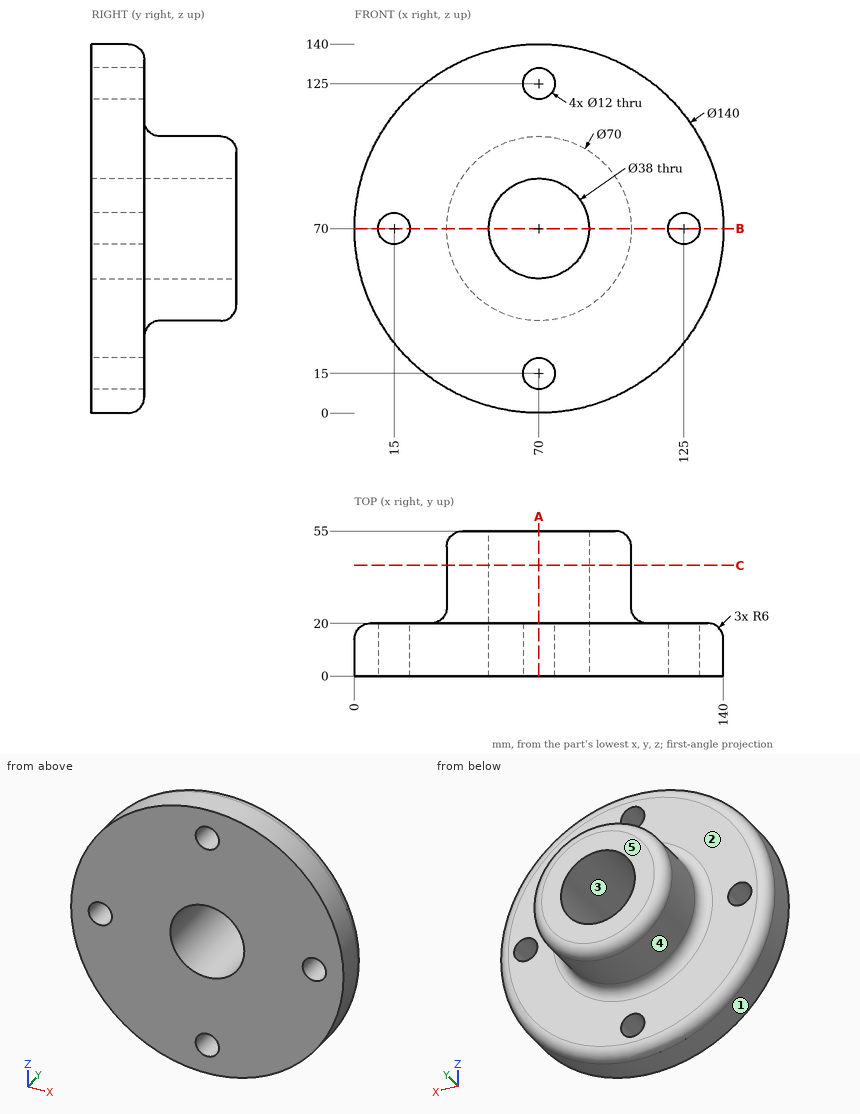
Could you check a few things on this drawing? It's one solid part, dimensions in mm from its lowest x, y, z. A direction names the side the tool comes from. Coordinates: 2 decimals unless noted, no trailing zeros. Loops run counter-clockwise (first coordinate to the right, second up) from the corner with the lowest first, then second, coordinate; pieces in that order, holes last. Notation, with made-up numbers: (67.5, -34.75) - (104.5, -34.75) arc R29 cw to (104.5, -2.75) - close; hole circle Ø7 at (-37, -37). An arc over 180 degrees is marked (long way). Answer as a JSON object with one key per item and string values. Group by question number.
Item 1: For pin 1 (9.5 mm diameter, centred on x = 125, z = 70, fed in from +Y); pin 2 (1.5 mm diameter, centred on x = 41, z = 47, fed in from +Y); pin 3 (2 mm diameter, centred on y = 10, z = 38.5, fed in from +X); pin 4 (2 mm diameter, centred on y = 13.5, z = 76, fed in from -X), each with a flat end and sliding along its axis, tell me the tip position at first contact or that it passes through.
Item 2: If I drill on L1, parallel to Z at x = 70, y = 12; L2, parallel to Z at x = 70, y = 38; L3, parallel to Y at x = 34, z = 119, over which ranges is the centre line in solid material (lowest first)? Write a range as from..to.
Item 3: If we section it at C-C (y = 42): List the corners of the cut face in (x, z) for me.
Item 4: On a 3-axis mill with a long thin cutter (end or side, diameter ignored), from which of +Z, -Z, +X, -X, +Y, -Y can I reach the whole of each face in a straight line? I mean the marked faces 4 and 5. Say none if no direction works.
Item 5: If we section it at B-B (z = 70): List the corners of the cut face in (x, y) for me.
Item 6: If we mould it in two halves opening along Z, with no side actions, what happens to the marked faces 1, 2 and 3? For each: released by +Z, released by -Z, zero draft, split by the parting line, or undercut.
Item 7: If we section it at A-A (x = 70): List the corners of the cut face in (y, z) for me.
Returned:
{
 "1": {"pin 1": "passes through", "pin 2": "stops at y = 22.32", "pin 3": "stops at x = 133.01", "pin 4": "stops at x = 0.18"},
 "2": {"L1": "z = 0..9, 21..51, 89..119, 131..140", "L2": "z = 35..51, 89..105", "L3": "y = 0..20"},
 "3": {"outline": "circle Ø70 at (70, 70); hole circle Ø38 at (70, 70)"},
 "4": {"face 4": "+Y", "face 5": "+Z, -Z, +X, -X, +Y"},
 "5": {"outline": "(0, 0) - (9, 0) - (9, 20) - (6, 20) arc R6 ccw to (0, 14) - close; (21, 0) - (51, 0) - (51, 55) - (41, 55) arc R6 ccw to (35, 49) - (35, 26) arc R6 cw to (29, 20) - (21, 20) - close; (89, 0) - (119, 0) - (119, 20) - (111, 20) arc R6 cw to (105, 26) - (105, 49) arc R6 ccw to (99, 55) - (89, 55) - close; (131, 0) - (140, 0) - (140, 14) arc R6 ccw to (134, 20) - (131, 20) - close"},
 "6": {"face 1": "split by the parting line", "face 2": "zero draft", "face 3": "undercut"},
 "7": {"outline": "(0, 0) - (14, 0) arc R6 ccw to (20, 6) - (20, 9) - (0, 9) - close; (0, 21) - (20, 21) - (20, 29) arc R6 cw to (26, 35) - (49, 35) arc R6 ccw to (55, 41) - (55, 51) - (0, 51) - close; (0, 89) - (55, 89) - (55, 99) arc R6 ccw to (49, 105) - (26, 105) arc R6 cw to (20, 111) - (20, 119) - (0, 119) - close; (0, 131) - (20, 131) - (20, 134) arc R6 ccw to (14, 140) - (0, 140) - close"}
}
